from build123d import *

# Parameters (mm, degrees)
SKETCH_1_W          = 2
SKETCH_1_H          = 2
EXTRUDE_1_DEPTH     = 3
EXTRUDE_2_DEPTH     = 124.5
SKETCH_3_W          = 6.103798984
SKETCH_3_H          = 7.216344691
CUT_EXTRUDE_1_DEPTH = 100
SKETCH_4_R          = 1
SKETCH_4_R_2        = 1.050016024
SKETCH_4_R_3        = 1.05
CUT_EXTRUDE_2_DEPTH = 100
SKETCH_6_W          = 76.933972046
SKETCH_6_H          = 147.245046369
CUT_EXTRUDE_3_DEPTH = 100
EXTRUDE_3_DEPTH     = 2
EXTRUDE_4_DEPTH     = 4
SKETCH_9_W          = 19.878498858
SKETCH_9_H          = 18.624082489
CUT_EXTRUDE_4_DEPTH = 4
SKETCH_10_W         = 19.878498858
SKETCH_10_H         = 38
CUT_EXTRUDE_5_DEPTH = 4
EXTRUDE_6_DEPTH     = 4
EXTRUDE_7_DEPTH     = 4
SKETCH_14_R         = 1.35
CUT_EXTRUDE_7_DEPTH = 4
SKETCH_15_R         = 1.35
CUT_EXTRUDE_8_DEPTH = 4


with BuildPart() as part:
    # 草图1 → 凸台-拉伸1 (new body)
    with BuildSketch(Plane(origin=(0, 0, 0), x_dir=(1, 0, 0), z_dir=(0, 1, 0))):
        Rectangle(SKETCH_1_W, SKETCH_1_H)
    extrude(amount=EXTRUDE_1_DEPTH)

    # 草图2 → 凸台-拉伸2 (add)
    with BuildSketch(Plane(origin=(0, 0, -1), x_dir=(-1, 0, 0), z_dir=(0, 0, -1))):
        Polygon((-9.439249429, 3), (10.439249429, 3), (31.447953726, 5.562037109), (31.447953726, 3.562037109), (10.439249429, 1), (-9.439249429, 1), (-30.447953726, 3.562037109), (-30.447953726, 5.562037109), align=None)
    extrude(amount=-EXTRUDE_2_DEPTH)

    # 草图3 → 切除-拉伸1 (cut)
    with BuildSketch(Plane.XZ.offset(-1)):
        with Locations((-0.416327581, 1.421882079)):
            Rectangle(SKETCH_3_W, SKETCH_3_H)
    extrude(amount=CUT_EXTRUDE_1_DEPTH, mode=Mode.SUBTRACT)

    # 草图4 → 切除-拉伸2 (cut)
    with BuildSketch(Plane.XZ.offset(-1)):
        with Locations(Location((24, 97.999988001, 0), (0, 0, 180))):
            Circle(SKETCH_4_R)
        with Locations(Location((6.500166, 99, 0), (0, 0, 270))):
            Circle(SKETCH_4_R)
        with Locations(Location((-7.499834, 99, 0), (0, 0, 270))):
            Circle(SKETCH_4_R)
        with Locations((-24.999894002, 97.999988001)):
            Circle(SKETCH_4_R)
        with Locations(Location((6.500166, 19, 0), (0, 0, 270))):
            Circle(SKETCH_4_R)
        with Locations(Location((-7.499834, 19, 0), (0, 0, 270))):
            Circle(SKETCH_4_R)
        with Locations(Location((24, 21.999986001, 0), (0, 0, 180))):
            Circle(SKETCH_4_R_2)
        with Locations((-24.999894002, 21.999986001)):
            Circle(SKETCH_4_R_3)
    extrude(amount=-CUT_EXTRUDE_2_DEPTH, mode=Mode.SUBTRACT)

    # 草图6 → 切除-拉伸3 (cut)
    with BuildSketch(Plane.XZ.offset(-1)):
        with Locations((-0.585190424, 56.41539679)):
            Rectangle(SKETCH_6_W, SKETCH_6_H)
        Polygon((-31.447953726, 18.875917511), (-14.439249429, 12.875917511), (-10.439249429, -1.124082489), (9.439249429, -1.124082489), (13.439249429, 12.875917511), (30.447953726, 18.875917511), (30.447953726, 26.875917511), (13.439249429, 29.875917511), (13.439249429, 87.875917511), (30.447953726, 93.875917511), (30.447953726, 101.875917511), (13.439249429, 104.875917511), (13.439249429, 123.5), (-14.439249429, 123.5), (-14.439249429, 104.875917511), (-31.329711994, 101.875917511), (-31.329711994, 93.875917511), (-14.439249429, 87.875917511), (-14.439249429, 29.875917511), (-31.447953726, 26.875917511), align=None, mode=Mode.SUBTRACT)
    extrude(amount=-CUT_EXTRUDE_3_DEPTH, mode=Mode.SUBTRACT)

    # 草图7 → 凸台-拉伸3 (add)
    with BuildSketch(Plane.XY.offset(123.5)):
        Polygon((-14.439249429, 1.487804878), (-10.439249429, 1), (-10.439249429, -12), (-14.439249429, -12), (-14.439249429, 1), align=None)
    extrude_3 = extrude(amount=-EXTRUDE_3_DEPTH)

    # 草图8 → 凸台-拉伸4 (add)
    with BuildSketch(Plane.ZY.offset(14.439249429)):
        Polygon((51.587761239, 1.487804878), (121.5, 1.487804878), (121.5, -12), (93.804336039, -12), (89.124737206, -6.169338891), align=None)
        Polygon((81.404880427, -0.512195122), (119.5, -0.512195122), (119.5, -8), (106.737581435, -8), (95.722961725, -8), (92.704938742, -4.239620134), (91.339916161, -2.53883672), align=None, mode=Mode.SUBTRACT)
    extrude_4 = extrude(amount=-EXTRUDE_4_DEPTH)

    # 草图9 → 切除-拉伸4 (cut)
    with BuildSketch(Plane(origin=(0, 3, 0), x_dir=(1, 0, 0), z_dir=(0, 1, 0))):
        with Locations((-0.5, -114.187958756)):
            Rectangle(SKETCH_9_W, SKETCH_9_H)
    cut_extrude_4 = extrude(amount=-CUT_EXTRUDE_4_DEPTH, mode=Mode.SUBTRACT)

    # 草图10 → 切除-拉伸5 (cut)
    with BuildSketch(Plane(origin=(0, 3, 0), x_dir=(1, 0, 0), z_dir=(0, 1, 0))):
        with Locations((-0.5, -58.875917511)):
            Rectangle(SKETCH_10_W, SKETCH_10_H)
    cut_extrude_5 = extrude(amount=-CUT_EXTRUDE_5_DEPTH, mode=Mode.SUBTRACT)

    # 草图11 → 凸台-拉伸6 (add)
    with BuildSketch(Plane.XZ.offset(12)):
        Polygon((-17.03732564, 97.222961725), (-14.439249429, 95.722961725), (-14.439249429, 101.722961725), (-17.03732564, 100.222961725), align=None)
        Polygon((-17.03732564, 113), (-14.439249429, 111.5), (-14.439249429, 117.5), (-17.03732564, 116), align=None)
    extrude_6 = extrude(amount=-EXTRUDE_6_DEPTH)

    # 草图13 → 凸台-拉伸7 (add)
    with BuildSketch(Plane.XY.offset(123.5)):
        Polygon((-14.439249429, -6.512195122), (-14.439249429, -0.512195122), (-17.03732564, -2.012195122), (-17.03732564, -5.012195122), align=None)
    extrude_7 = extrude(amount=-EXTRUDE_7_DEPTH)

    # 草图14 → 切除-拉伸7 (cut)
    with BuildSketch(Plane.XY.offset(123.5)):
        with Locations((-14.439249429, -3.512195122)):
            Circle(SKETCH_14_R)
    cut_extrude_7 = extrude(amount=-CUT_EXTRUDE_7_DEPTH, mode=Mode.SUBTRACT)

    # 草图15 → 切除-拉伸8 (cut)
    with BuildSketch(Plane.XZ.offset(12)):
        with Locations(Location((-14.439249429, 98.722961725, 0), (0, 0, 270))):
            Circle(SKETCH_15_R)
        with Locations(Location((-14.439249429, 114.5, 0), (0, 0, 270))):
            Circle(SKETCH_15_R)
    cut_extrude_8 = extrude(amount=-CUT_EXTRUDE_8_DEPTH, mode=Mode.SUBTRACT)

    # 镜向1: 凸台-拉伸3, 凸台-拉伸4, 切除-拉伸4, 切除-拉伸5, 凸台-拉伸6, 凸台-拉伸7, 切除-拉伸7, 切除-拉伸8 across plane
    add(extrude_3.mirror(Plane.ZY.offset(0.5)))
    add(extrude_4.mirror(Plane.ZY.offset(0.5)))
    add(cut_extrude_4.mirror(Plane.ZY.offset(0.5)), mode=Mode.SUBTRACT)
    add(cut_extrude_5.mirror(Plane.ZY.offset(0.5)), mode=Mode.SUBTRACT)
    add(extrude_6.mirror(Plane.ZY.offset(0.5)))
    add(extrude_7.mirror(Plane.ZY.offset(0.5)))
    add(cut_extrude_7.mirror(Plane.ZY.offset(0.5)), mode=Mode.SUBTRACT)
    add(cut_extrude_8.mirror(Plane.ZY.offset(0.5)), mode=Mode.SUBTRACT)


solid = part.part
Geometry check sheet. Reference: the model listing, model coordinates, mm. A direction names the side the tool comes from. Give positions to 0.01 mm unless a question says otherwise; leave off trailing zeros. Loops run counter-clockwise (first coordinate to the right, second up) from the corner with the lowest first, then second, coordinate; pieces in that order, holes last. Notation, with made-up numbers: (48.5, 8) -> (62.5, 8) arc R12 ccw to (62.5, 14) -> close; hole circle Ø10 at (30, 16). An arc over 180 degrees is marked (long way). Answer in a Markdown table with one row per item. Add a question column.
1) Material ranges on probe 1 along X at (y, z) = (-10.25, 103.5); probe 2 along Z at (x, y) = (-26.5, 4.5); probe 3 along Y at (x, z) = (-3.5, 27), recorded low to high. Write a range as from..to.
2) Cross-section at B-B on z = 114.5. Record the boundary of the cut face in (x, y).
3) Cross-section at A-A on x = 0. Record the boundary of the cut face in (y, z).
4) Cross-section at C-C on y = -10.75. Record the boundary of the cut face in (x, z).
5) Draft check along Y on faces 1 (the face through (-18.756, 2.014, 26.105)), 2 (the face through (-13.15, -3.11, 121.53)), 3 (the face through (14.72, -1.25, 121.53)), 4 (the face through (14.756, -10.028, 112.26)). Enter one of: pulls with the +Y half, pulls with the -Y half, needs draft (parallel to the pull), parting line crosses it, or undercut.
6) Set-up check for faces 5 (the face through (0, 3, 91)), 6 (the face through (-13, -8, 108)), 7 (the face through (14.756, -10.028, 96.483)): record each of +Z, -Z, +X, -X, +Y, -Y from which the full face is reachable in a straight line by a thin tool's end or side.
7) Gauge pin test, flat ends, axial feed: P1, Ø8, axis at y = -1, z = 72, coming from the +X side; P2, Ø0.9, axis at y = -4, z = 122, coming from the +X side; P3, Ø4, axis at x = -8.5, z = 83, coming from the +Y side. Record the tip position at first contact, or that the pin passes through.
Outcome:
| question | item | result |
|---|---|---|
| 1 | probe 1 | x = -14.44..-10.44, 9.44..13.44 |
| 1 | probe 2 | z = 17.13..27.75, 92.16..102.73 |
| 1 | probe 3 | y = 1..3 |
| 2 | outline | (-17.04, -12) -> (-15.79, -12) -> (-15.79, -8) -> (-17.04, -8) -> close; (-14.44, -0.51) -> (-10.44, -0.51) -> (-10.44, 3) -> (-14.44, 3.49) -> close; (-13.09, -12) -> (-10.44, -12) -> (-10.44, -8) -> (-13.09, -8) -> close; (9.44, -12) -> (12.09, -12) -> (12.09, -8) -> (9.44, -8) -> close; (9.44, -0.51) -> (13.44, -0.51) -> (13.44, 3.49) -> (9.44, 3) -> close; (14.79, -12) -> (16.04, -12) -> (16.04, -8) -> (14.79, -8) -> close |
| 3 | outline | (1, -1) -> (3, -1) -> (3, 39.88) -> (1, 39.88) -> close; (1, 77.88) -> (3, 77.88) -> (3, 104.88) -> (1, 104.88) -> close |
| 4 | outline | (-17.04, 97.22) -> (-14.44, 95.72) -> (-14.44, 92.8) -> (-10.44, 92.8) -> (-10.44, 123.5) -> (-14.44, 123.5) -> (-14.44, 117.5) -> (-17.04, 116) -> (-17.04, 113) -> (-14.44, 111.5) -> (-14.44, 101.72) -> (-17.04, 100.22) -> close; (9.44, 92.8) -> (13.44, 92.8) -> (13.44, 95.72) -> (16.04, 97.22) -> (16.04, 100.22) -> (13.44, 101.72) -> (13.44, 111.5) -> (16.04, 113) -> (16.04, 116) -> (13.44, 117.5) -> (13.44, 123.5) -> (9.44, 123.5) -> close; hole circle Ø2.7 at (-14.44, 98.72); hole circle Ø2.7 at (-14.44, 114.5); hole circle Ø2.7 at (13.44, 98.72); hole circle Ø2.7 at (13.44, 114.5) |
| 5 | face 1 | pulls with the -Y half |
| 5 | face 2 | undercut |
| 5 | face 3 | pulls with the +Y half |
| 5 | face 4 | needs draft |
| 6 | face 5 | +Z, -Z, +Y |
| 6 | face 6 | +X, -X |
| 6 | face 7 | -Z, +X, -Y |
| 7 | P1 | stops at x = 13.44 |
| 7 | P2 | stops at x = 16.04 |
| 7 | P3 | stops at y = 3.01 |
